Design review of the part shown in the three views and the two pictorial views. Dimensions are in mm from the part's minimum x, y and z. A direction names the side the tool comes from. Give positions to 0.01 mm unless a question says otherwise; leave off trailing zeros. Order: outer loops, then holes, each group sorted by start corner. A loop starts at its lowest first (then second) coordinate and runs counter-clockwise, first axis right, second up.
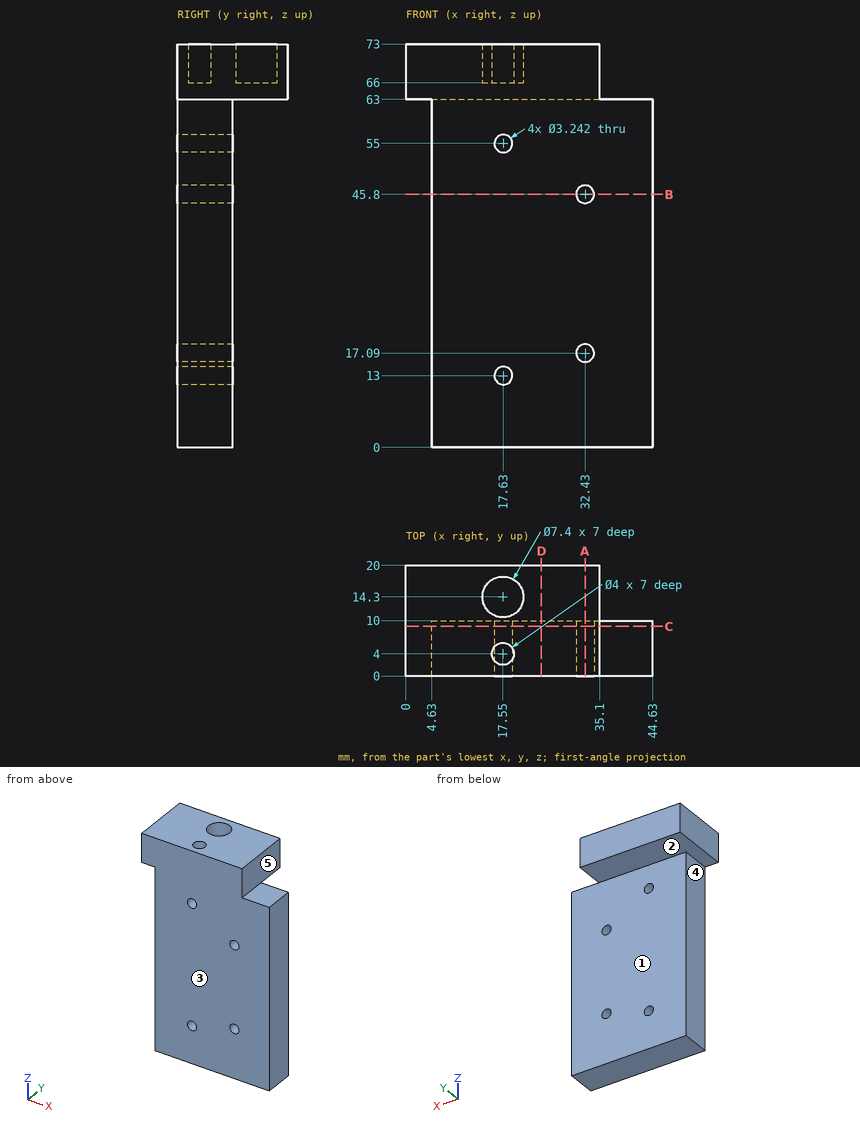
Item 1: Take a section at B-B (z = 45.8). Give the boundary of the cut face in (x, y), and give its area (3 significant figures).
Values found:
outline: (4.63, 0) - (30.81, 0) - (30.81, 10) - (4.63, 10) - close; (34.05, 0) - (44.63, 0) - (44.63, 10) - (34.05, 10) - close
area: 368 mm2
Item 2: For line 1 (Z direction, x = 32.43, y = 4.5); line 2 (Y direction, x = 17, z = 70); line 3 (X direction, y = 4, z = 45.8), list the stretches that pass through material, from the lowest coordinate up.
Values found:
line 1: z = 0 to 15.47, 18.71 to 44.18, 47.42 to 73
line 2: y = 0 to 2.08, 5.92 to 10.64, 17.96 to 20
line 3: x = 4.63 to 30.81, 34.05 to 44.63
Item 3: Take a section at A-A (x = 32.43). Give the boundary of the cut face in (y, z), and give its area (3 significant figures).
Values found:
outline: (0, 0) - (10, 0) - (10, 15.47) - (0, 15.47) - close; (0, 18.71) - (10, 18.71) - (10, 44.18) - (0, 44.18) - close; (0, 47.42) - (10, 47.42) - (10, 63) - (20, 63) - (20, 73) - (0, 73) - close
area: 765 mm2
Item 4: For the marked faces 1, 2, 3, 4 and 5, list the 3-axis set-ups (+Z, -Z, +X, -X, +Y, -Y) from which the entire face can be reached by the end or side of a thin tool; tool diameter is ignored.
Values found:
face 1: -Z, +X, -X, +Y
face 2: -Z, -X, +Y
face 3: +Z, -Z, +X, -X, -Y
face 4: -Z, -X, +Y, -Y
face 5: +Z, +X, +Y, -Y
Item 5: Take a section at C-C (y = 9). Give the boundary of the cut face in (x, z), and give its area (3 significant figures).
Values found:
outline: (0, 63) - (4.63, 63) - (4.63, 0) - (44.63, 0) - (44.63, 63) - (35.1, 63) - (35.1, 73) - (0, 73) - close; hole circle Ø3.24 at (17.63, 13); hole circle Ø3.24 at (17.63, 55); hole circle Ø3.24 at (32.43, 17.09); hole circle Ø3.24 at (32.43, 45.8)
area: 2,840 mm2
Item 6: Clearance check with flat-ended pins moving along their axes: pin 1 Ø2 at (x, y) = (19, 15) entering from +Z; pin 2 Ø12 at (x, y) = (40, 18) entering from -Z; pin 3 Ø3 at (x, z) = (25, 53) entering from +Y. State where each tip first meets the part, or that it passes through.
Values found:
pin 1: stops at z = 66
pin 2: stops at z = 63
pin 3: stops at y = 10
Item 7: Take a section at D-D (x = 24.5). Give the boundary of the cut face in (y, z).
Values found:
outline: (0, 0) - (10, 0) - (10, 63) - (20, 63) - (20, 73) - (0, 73) - close
